Autodesk Inventor part; units mm, degrees
ref_plane "YZ Plane" through (0, 0, 0) normal (1, 0, 0) x (0, 1, 0)
ref_plane "XZ Plane" through (0, 0, 0) normal (0, 1, 0) x (-1, 0, 0)
ref_plane "XY Plane" through (0, 0, 0) normal (0, 0, 1) x (1, 0, 0)
sketch "Sketch1" plane through (0, 0, 0) normal (0, 1, 0) x (-1, 0, 0)
  line L0 (0, 0) -> (0, -59.5)
  line L1 (0, -59.5) -> (3, -59.5)
  line L2 (3, -59.5) -> (3, -54.5)
  line L3 (3, -54.5) -> (39, -54.5)
  line L4 (39, -54.5) -> (39, -52)
  line L5 (39, -52) -> (3, -52)
  line L6 (3, -52) -> (3, 0)
  line L7 (3, 0) -> (0, 0)
  dimension "d3" = 3
  dimension "d4" = 5
  dimension "d5" = 36
  dimension "d6" = 2.5
  dimension "d14" = 52
revolve "Revolution1" add sketch "Sketch1" angle 360 about axis through (-3, 0, 0) along (1, 0, 0)
chamfer "Chamfer1" distance 2 angle 45 1 edges at (-39, 0, 54.5)
sketch "Sketch4" plane through (0, 0, 0) normal (1, 0, 0) x (0, 0, -1)
  line L0 (-25, -25) -> (25, -25)
  line L1 (25, -25) -> (25, 25)
  line L2 (25, 25) -> (-25, 25)
  line L3 (-25, 25) -> (-25, -25)
  line L4 (-25, -25) -> (25, 25) construction
  line L5 (25, -25) -> (-25, 25) construction
  point P0 (0, 0)
  point P1 (0, 0)
  dimension "d20" = 50
extrude "Extrusion3" cut sketch "Sketch4" against normal blind 10
properties part number "aftPlug" material "PVC-Piping"
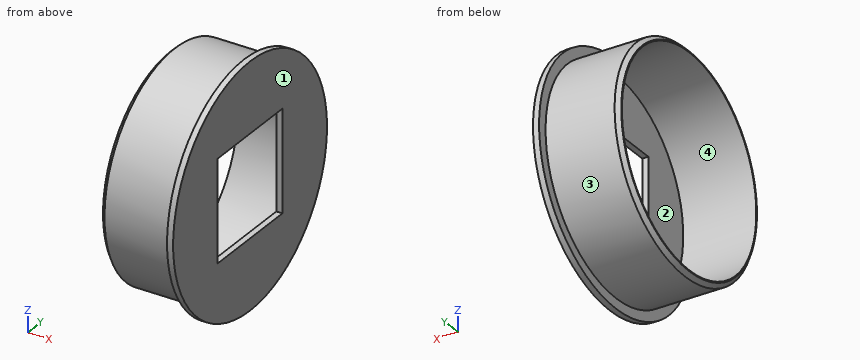
For this review, take the finished solid that the model builds, in its own axes (mm). Face numbers are marked on the shaded views. Round coordinates to 2 decimals unless told otherwise and drop trailing zeros. Write each loop counter-clockwise with the first axis right and the second up, starting at its lowest first coordinate (ties: lowest second). Pieces come first, ordered by that corner, then holes.
1) Insertion check: pin 1 Ø0.9 at (x, y) = (-2, -11.5) entering from +Z; pin 2 Ø6 at (x, y) = (-18, 0) entering from -Z; pin 3 Ø8 at (x, y) = (-14, -1) entering from +Z. Each pin has a flat end and moves straight along its axis. Give the tip position at first contact, or say it passes through.
Answer below:
pin 1: stops at z = 58.46
pin 2: stops at z = -54.5
pin 3: stops at z = 54.5
2) Take a section at C-C on x = -8. Give the boundary of the cut face in (y, z), then the cut area to 3 significant figures.
Answer below:
outline: circle Ø109 at (0, 0); hole circle Ø104 at (0, 0)
area: 836 mm2
3) Mouldability with a two-part tool opening along Z and no side actions: class the marked faces 1, 2, 3 and 4 as +Z half, -Z half, draft (parallel to the pull), parting line (faces both ways), or undercut.
Answer below:
face 1: draft
face 2: undercut
face 3: parting line
face 4: undercut
4) Take a section at A-A on z = 0. Give the boundary of the cut face in (x, y).
Answer below:
outline: (-39, -52.5) - (-37, -54.5) - (-3, -54.5) - (-3, -59.5) - (0, -59.5) - (0, -25) - (-3, -25) - (-3, -52) - (-39, -52) - close; (-39, 52) - (-3, 52) - (-3, 25) - (0, 25) - (0, 59.5) - (-3, 59.5) - (-3, 54.5) - (-37, 54.5) - (-39, 52.5) - close
5) For line 1 along Y through (x, z) = (-30, 0); line 2 along X through (y, z) = (44, 25); line 3 along Z through (x, y) = (-6, 3.5), list the stretches that pass through material, from the lowest coordinate up.
Answer below:
line 1: y = -54.5 to -52, 52 to 54.5
line 2: x = -3 to 0
line 3: z = -54.39 to -51.88, 51.88 to 54.39
